Source: three-view drawing plus pictorial views. Frame: mm from the lowest corner of the part. A direction names the side the tool comes from. Coordinates: 2 decimals unless noted, no trailing zeros. Order: outer loops, then holes, each group sorted by start corner. A loop starts at its lowest first (then second) coordinate and runs counter-clockwise, first axis right, second up. Notation, with made-up numbers: (-19, 45) - (21, 45) arc R28 ccw to (21, 73) - close; hole circle Ø8 at (0.25, -6.5). An arc over 180 degrees is marked (long way). One line per question, with ' | ' between items.
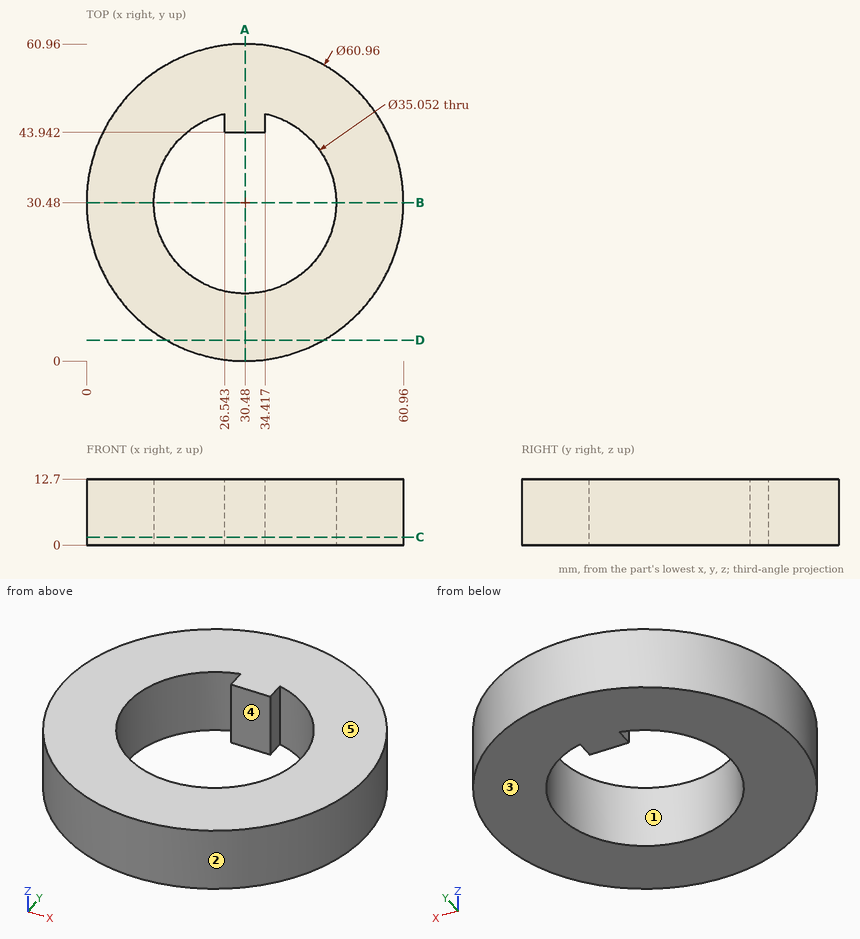
Item 1: Section A-A on x = 30.48. Return the cut outline in (y, z).
Data:
outline: (0, 0) - (12.95, 0) - (12.95, 12.7) - (0, 12.7) - close; (43.94, 0) - (60.96, 0) - (60.96, 12.7) - (43.94, 12.7) - close
Item 2: Section B-B on y = 30.48. Return the cut outline in (x, z).
Data:
outline: (0, 0) - (12.95, 0) - (12.95, 12.7) - (0, 12.7) - close; (48.01, 0) - (60.96, 0) - (60.96, 12.7) - (48.01, 12.7) - close
Item 3: Access query for the marked faces 4 and 5. Directions: +Z, -Z, +X, -X, +Y, -Y. A direction counts if a zero-diameter tool reaches every point of the face in a straight line with its end or side. Return the directions, or none.
Data:
face 4: +Z, -Z | face 5: +Z, +X, -X, +Y, -Y
Item 4: Section D-D on y = 4. Return the cut outline in (x, z), and give its area (3 significant figures).
Data:
outline: (15.39, 0) - (45.57, 0) - (45.57, 12.7) - (15.39, 12.7) - close | area: 383 mm^2
Item 5: Draft query along X for the marked faces 1, 2 and 3. Return one class per face: released by +X, released by -X, zero draft, split by the parting line, or undercut.
Data:
face 1: undercut | face 2: split by the parting line | face 3: zero draft
Item 6: Section C-C on z = 1.5. Return the cut outline in (x, y).
Data:
outline: circle Ø60.96 at (30.48, 30.48); hole (26.54, 43.94) - (26.54, 47.56) arc R17.53 ccw (long way) to (34.42, 47.56) - (34.42, 43.94) - close
Item 7: Ray query, line 1 (Y direction, x = 30.48, z = 5.75); line 2 (X direction, y = 30, z = 2); line 3 (Y direction, x = 28.5, z = 7.25). Return the intervals inside material, ascending.
Data:
line 1: 0 to 12.95, 43.94 to 60.96 | line 2: 0 to 12.96, 48 to 60.96 | line 3: 0.06 to 13.07, 43.94 to 60.9
Item 8: Contact query for flat-ended pins moving along their axis: P1, Ø1.5, axis at x = 50, z = 10.5, coming from the -Y side; P2, Ø1.5, axis at x = 41, z = 11, coming from the +Y side; P3, Ø1.1, axis at y = 46, z = 9, coming from the +X side. Output: stop coordinate, or through.
Data:
P1: y = 6.47 | P2: y = 59.35 | P3: x = 57.03
